The drawing under review shows one solid part. Ordinate dimensions are in mm from its lowest x, y, z. A direction names the side the tool comes from. Give positions to 0.01 mm unless a question says otherwise; leave off trailing zeros. Order: outer loops, then holes, each group sorted by start corner. A loop starts at its lowest first (then second) coordinate and runs counter-clockwise, first axis right, second up. Notation, with made-up numbers: (-32, 40) - (12, 40) arc R22 ccw to (12, 76) - close; hole circle Ø4 at (81.5, 70). An arc over 180 degrees is marked (long way). Write item = value, one per line. Start each with the question number.
1. Wall thickness on probe 1 along X at (y, z) = (32.5, 22); probe 2 along X at (y, z) = (2, 22); probe 3 along Y at (x, z) = (16, 30.5): over which ranges is each line inside the solid? List them lowest first.
2. Machinability: for the marked faces 4 and 5, which of the approach directions +Z, -Z, +X, -X, +Y, -Y give a long, thin tool a straight path to every point of the face, cutting with its end or side? Answer none if there is none.
3. We need section B-B, the plane x = 22. Give the boundary of the cut face in (y, z).
4. Mouldability with a two-part tool opening along X and no side actions: class the marked faces 1, 2 and 3 as pulls with the +X half, pulls with the -X half, needs draft (parallel to the pull), parting line crosses it, or undercut.
5. We need section A-A, the plane z = 22. Give the boundary of the cut face in (x, y).
6. We need section C-C, the plane y = 23. Give the boundary of the cut face in (x, z).
7. We need section D-D, the plane z = 10. Give the boundary of the cut face in (x, y), and give its area (3 significant figures).
8. For P1, Ø15, axis at x = 23, z = 28, coming from the -Y side; P2, Ø5, axis at x = 12.5, y = 8.5, coming from the +Z side; P3, Ø6, axis at x = 14, y = 11, coming from the +Z side, all flat-tipped, find the tip position at first contact; note any pin that passes through.
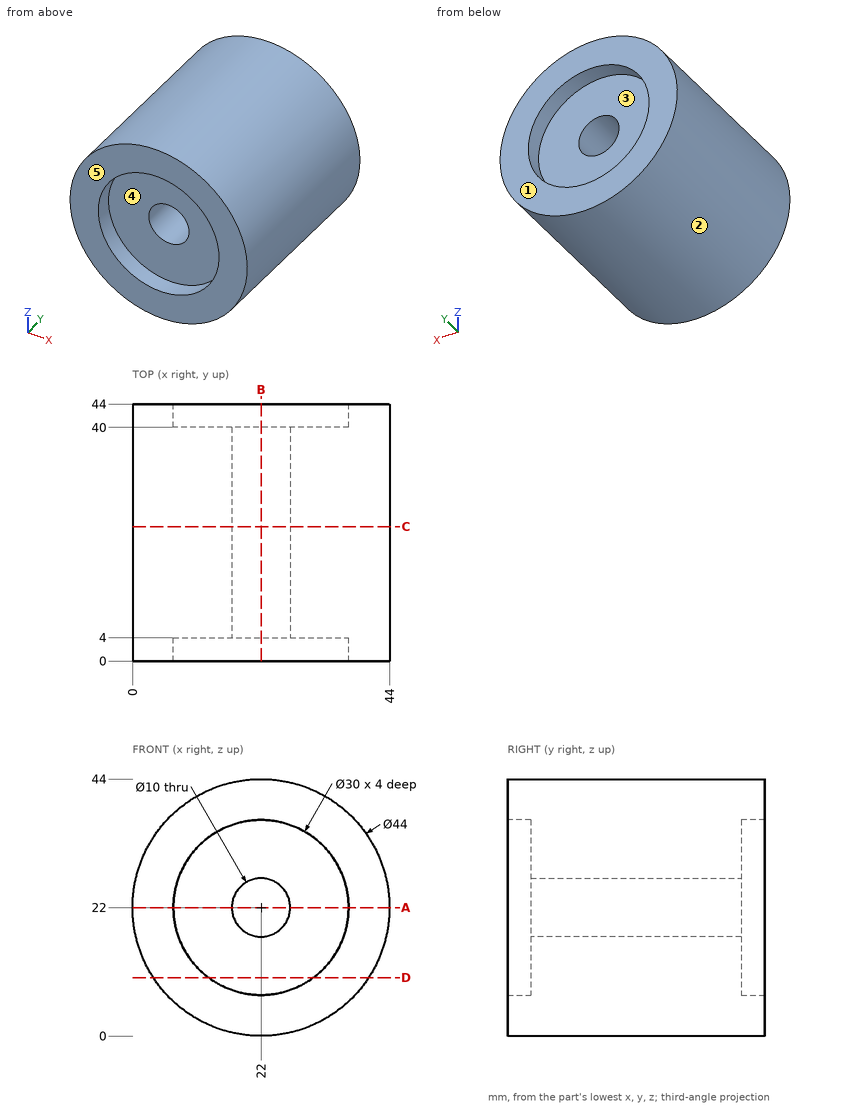
Model answer:
q1.probe_1 = 0 to 17, 27 to 44
q1.probe_2 = 0 to 7, 37 to 44
q1.probe_3 = 4 to 40
q2.face_4 = -Y
q2.face_5 = +Z, -Z, +X, -X, -Y
q3.outline = (0, 0) - (44, 0) - (44, 7) - (40, 7) - (40, 17) - (4, 17) - (4, 7) - (0, 7) - close; (0, 37) - (4, 37) - (4, 27) - (40, 27) - (40, 37) - (44, 37) - (44, 44) - (0, 44) - close
q4.face_1 = needs draft
q4.face_2 = parting line crosses it
q4.face_3 = undercut
q5.outline = (0, 0) - (7, 0) - (7, 4) - (17, 4) - (17, 40) - (7, 40) - (7, 44) - (0, 44) - close; (27, 4) - (37, 4) - (37, 0) - (44, 0) - (44, 44) - (37, 44) - (37, 40) - (27, 40) - close
q6.outline = circle Ø44 at (22, 22); hole circle Ø10 at (22, 22)
q7.outline = (3.56, 0) - (13, 0) - (13, 4) - (31, 4) - (31, 0) - (40.44, 0) - (40.44, 44) - (31, 44) - (31, 40) - (13, 40) - (13, 44) - (3.56, 44) - close
q7.area = 1,480 mm2
q8.P1 = 4
q8.P2 = 42.86
q8.P3 = 43.42
